Design review of the part built by this model. Coordinates are the model's own, in mm. Coordinates: 2 decimals unless noted, no trailing zeros. Write each loop counter-clockwise with the first axis right and the second up, starting at its lowest first coordinate (ties: lowest second). Pieces come first, ordered by that corner, then holes.
Q1. Add section D-D, the plane y = 1.2. Give the boundary of the cut face in (x, z) (3 decimals), plus the area to 3 significant figures.
Q2. To check wall thickness, follow probe 1 along X at (y, z) = (2.2, -6.35); probe 2 along X at (y, z) = (1.55, -6.35); probe 3 along X at (y, z) = (2.75, -11.25). State the ranges of each line that lie inside material, in increasing order.
Q3. Add section B-B, the plane y = 2.7. Give the boundary of the cut face in (x, z) (3 decimals), plus the area to 3 significant figures.
Q4. Clearance check with a flat-ended pin moving along its axis: pin 1 Ø1 at (y, z) = (1, -4.5) entering from +X. State where the tip first meets the part, or that it passes through.
Q5. The part is to be moulded in two halves that separate along X. For faces 1 (the face through (2, 2, -6)), 2 (the face through (9.38, 1.61, -7.47)), 3 (the face through (9, 0, -5)), say which applies: +X half, -X half, draft (parallel to the pull), parting line (faces both ways), or undercut.
from build123d import *

# Parameters (mm, degrees)
SKETCH1_W                 = 19.05
SKETCH1_H                 = 12.7
BOSS_EXTRUDE1_DEPTH       = 3.175
CHAMFER1_SIZE             = 3.175
TAP_DRILL_FOR_4_40_TAP1_D = 2.2606


with BuildPart() as part:
    # Sketch1 → Boss-Extrude1 (new body)
    with BuildSketch(Plane(origin=(0, 0, 0), x_dir=(1, 0, 0), z_dir=(0, 1, 0))):
        with Locations((9.525, 6.35)):
            Rectangle(SKETCH1_W, SKETCH1_H)
    extrude(amount=BOSS_EXTRUDE1_DEPTH)

    # Chamfer1
    chamfer1_edges = [part.edges().sort_by_distance(p)[0] for p in [
        (19.05, 3.175, -6.35),
        (0, 3.175, -6.35),
    ]]
    chamfer(chamfer1_edges, length=CHAMFER1_SIZE - 0.0001)  # a hair under: the kernel refuses the full size

    # Tap Drill for #4-40 Tap1 (through all)
    with Locations(Plane(origin=(0, 0, 0), x_dir=(-1, 0, 0), z_dir=(0, -1, 0))):
        with Locations((-9.525, 6.35)):
            Hole(TAP_DRILL_FOR_4_40_TAP1_D / 2)


solid = part.part
Here are the results:
1. outline: (1.2, -12.7) - (17.85, -12.7) - (17.85, 0) - (1.2, 0) - close; hole circle Ø2.261 at (9.525, -6.35)
1. area: 207 mm2
2. probe 1: x = 2.2 to 8.39, 10.66 to 16.85
2. probe 2: x = 1.55 to 8.39, 10.66 to 17.5
2. probe 3: x = 2.75 to 16.3
3. outline: (2.7, -12.7) - (16.35, -12.7) - (16.35, 0) - (2.7, 0) - close; hole circle Ø2.261 at (9.525, -6.35)
3. area: 169 mm2
4. pin 1: stops at x = 18.55
5. face 1: -X half
5. face 2: undercut
5. face 3: draft
